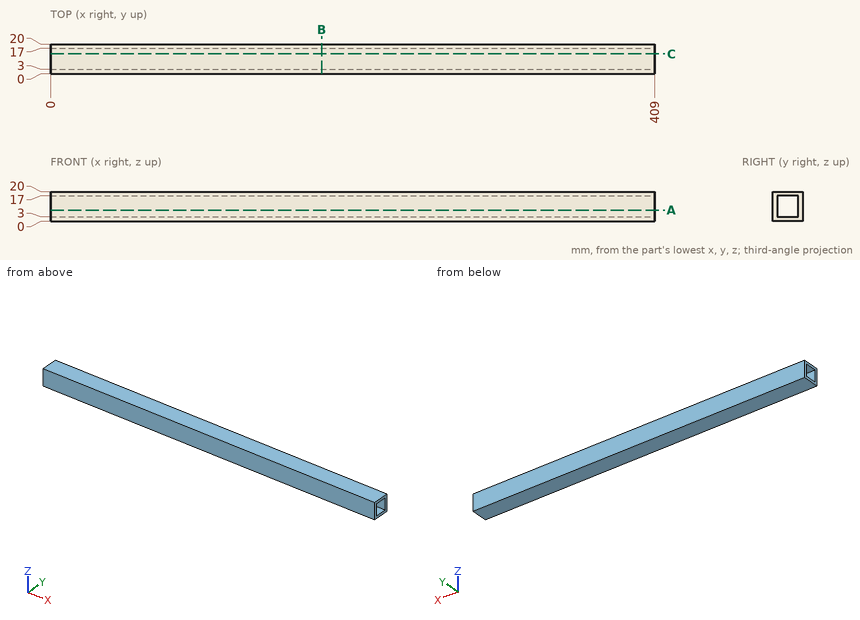
Source: three-view drawing plus pictorial views. Frame: mm from the lowest corner of the part. Give positions to 0.01 mm unless a question says otherwise; leave off trailing zeros. Write each loop counter-clockwise with the first axis right and the second up, starting at its lowest first coordinate (ties: lowest second). Pieces come first, ordered by that corner, then holes. Notation, with made-up numbers: (26, 36) - (75, 36) arc R16 cw to (75, 49) - close; hole circle Ø3 at (75, -19.5). An arc over 180 degrees is marked (long way). Write item = value, one per line. Start each with the question number.
Q1. Cut plane B-B, the plane x = 183.5. Return loops of the section in (y, z), then the cut area to 3 significant figures.
Q2. Cut plane A-A, the plane z = 7.5. Return loops of the section in (x, y), then the cut area to 3 significant figures.
Q3. Material intervals for probe 1 along Y at (x, z) = (332, 8.25), sorted ascending.
Computed values:
q1.outline = (0, 0) - (20, 0) - (20, 20) - (0, 20) - close; hole (3, 3) - (17, 3) - (17, 17) - (3, 17) - close
q1.area = 204 mm²
q2.outline = (0, 0) - (409, 0) - (409, 3) - (0, 3) - close; (0, 17) - (409, 17) - (409, 20) - (0, 20) - close
q2.area = 2,450 mm²
q3.probe_1 = 0 to 3, 17 to 20
